Can you work these out from the model? Positions are in its coordinate system, mm. Give positions to 0.01 mm unless a question says otherwise; leave off trailing zeros. Write each loop counter-clockwise with the first axis right and the second up, starting at its lowest first coordinate (ties: lowest second). Pieces come first, ordered by that corner, then holes.
```python
from build123d import *

# Parameters (mm, degrees)
BOSS_EXTRUDE1_DEPTH = 3.175


with BuildPart() as part:
    # Sketch1 → Boss-Extrude1 (new body, symmetric)
    with BuildSketch(Plane(origin=(0, 0, 0), x_dir=(0, 0, -1), z_dir=(1, 0, 0))):
        Polygon((0, 0), (0, 203.2), (24.3586, 203.2), (119.6086, 50.8), (24.3586, 0), align=None)
    extrude(amount=BOSS_EXTRUDE1_DEPTH, both=True)


solid = part.part
```
1) Suppose I cut it at A-A on x = 1.5. Write out the boundary of the cut face in (y, z), plus the area to 3 significant figures.
Values follow:
outline: (0, -24.36) - (50.8, -119.61) - (203.2, -24.36) - (203.2, 0) - (0, 0) - close
area: 14,600 mm2
2) For pin 1 Ø1 at (x, y) = (-0.5, 128) entering from -Z; pin 2 Ø2 at (x, y) = (0.5, 106) entering from -Z; pin 3 Ø2 at (x, z) = (-1.5, -45) entering from +Y, each with a flat end and sliding along its axis, tell me the tip position at first contact or that it passes through.
Values follow:
pin 1: stops at z = -71.67
pin 2: stops at z = -85.73
pin 3: stops at y = 171.77
3) Please list where these lines run through material, in increasing order: L1, parallel to Y at x = 2, z = -30; L2, parallel to Z at x = 0.5, y = 74; L3, parallel to Z at x = -1.75, y = 89.
Values follow:
L1: y = 3.01 to 194.17
L2: z = -105.11 to 0
L3: z = -95.73 to 0
4) Suppose I cut it at B-B on z = -47.5. Write out the boundary of the cut face in (x, y) (3 decimals), plus the area to 3 significant figures.
Values follow:
outline: (-3.175, 12.342) - (3.175, 12.342) - (3.175, 166.174) - (-3.175, 166.174) - close
area: 977 mm2
5) Suppose I cut it at C-C on y = 55. Write out the boundary of the cut face in (x, z) (3 decimals), plus the area to 3 significant figures.
Values follow:
outline: (-3.175, -116.984) - (3.175, -116.984) - (3.175, 0) - (-3.175, 0) - close
area: 743 mm2
